Can you work these out from the model? Positions are in its coordinate system, mm. Face numbers are marked on the shaded views. A direction names the side the tool comes from. Give positions to 0.01 mm unless a question says otherwise; leave off trailing zeros. Loops run counter-clockwise (first coordinate to the right, second up) from the corner with the lowest first, then second, coordinate; pieces in that order, holes last. Notation, with made-up numbers: (47, 58.25) - (70, 58.25) arc R15 ccw to (70, 85.25) - close; hole circle Ø2 at (16.25, 34). An arc over 180 degrees is marked (long way). Answer as a JSON object with one key per item and string values.
```python
from build123d import *

# Parameters (mm, degrees)
HEXAGON_DEPTH            = 5
SKETCH3_R                = 2
SCREW_POST_DEPTH         = 11
SKETCH4_R                = 2.5
BEARING_SECTION_DEPTH    = 14
SKETCH5_R                = 6.75
U_JOINT_BASE_DEPTH       = 3
U_JOINT_STANDUPS_DEPTH   = 9.5
STANDUP_ROUND_DEPTH      = 7.928203
STANDUP_ROUND_DEPTH_BACK = 7.928203
SKETCH8_R                = 1
BALL_HOLES_DEPTH         = 7.928203
BALL_HOLES_DEPTH_BACK    = 7.928203


with BuildPart() as part:
    # Sketch2 → Hexagon (new body)
    with BuildSketch(Plane.XY):
        Polygon((3.464102, -6), (6.928203, 0), (3.464102, 6), (-3.464102, 6), (-6.928203, 0), (-3.464102, -6), align=None)
    extrude(amount=HEXAGON_DEPTH)

    # Sketch3 → Screw Post (add)
    with BuildSketch(Plane.XY.offset(5)):
        Circle(SKETCH3_R)
    extrude(amount=SCREW_POST_DEPTH)

    # Sketch4 → Bearing Section (add)
    with BuildSketch(Plane(origin=(0, 0, 0), x_dir=(-1, 0, 0), z_dir=(0, 0, -1))):
        Circle(SKETCH4_R)
    extrude(amount=BEARING_SECTION_DEPTH)

    # Sketch5 → U Joint Base (add)
    with BuildSketch(Plane(origin=(0, 0, -14), x_dir=(-1, 0, 0), z_dir=(0, 0, -1))):
        Circle(SKETCH5_R)
    extrude(amount=U_JOINT_BASE_DEPTH)

    # Sketch6 → U Joint Standups (add)
    with BuildSketch(Plane(origin=(0, 0, -17), x_dir=(-1, 0, 0), z_dir=(0, 0, -1))):
        with BuildLine():
            Line((-5.771698, 3.5), (-3.75, 3.5))
            Line((-3.75, 3.5), (-3.75, -3.5))
            Line((-3.75, -3.5), (-5.771698, -3.5))
            ThreePointArc((-5.771698, -3.5), (-6.75, 0), (-5.771698, 3.5))
        make_face()
        with BuildLine():
            Line((3.75, -3.5), (3.75, 3.5))
            Line((3.75, 3.5), (5.771698, 3.5))
            ThreePointArc((5.771698, 3.5), (6.75, 0), (5.771698, -3.5))
            Line((5.771698, -3.5), (3.75, -3.5))
        make_face()
    extrude(amount=U_JOINT_STANDUPS_DEPTH)

    # Sketch7 → Standup Round (cut, two sides)
    with BuildSketch(Plane(origin=(0, 0, 0), x_dir=(0, 0, -1), z_dir=(1, 0, 0))) as standup_round_sk:
        with BuildLine():
            Line((26.5, -3.5), (26.5, 0))
            ThreePointArc((26.5, 0), (25.474874, -2.474874), (23, -3.5))
            Line((23, -3.5), (26.5, -3.5))
        make_face()
        with BuildLine():
            Line((26.5, 3.5), (23, 3.5))
            ThreePointArc((23, 3.5), (25.474874, 2.474874), (26.5, 0))
            Line((26.5, 0), (26.5, 3.5))
        make_face()
    extrude(amount=STANDUP_ROUND_DEPTH, mode=Mode.SUBTRACT)
    extrude(standup_round_sk.sketch, amount=-STANDUP_ROUND_DEPTH_BACK, mode=Mode.SUBTRACT)

    # Sketch8 → Ball Holes (cut, two sides)
    with BuildSketch(Plane(origin=(0, 0, 0), x_dir=(0, 0, -1), z_dir=(1, 0, 0))) as ball_holes_sk:
        with Locations((23, 0)):
            Circle(SKETCH8_R)
    extrude(amount=BALL_HOLES_DEPTH, mode=Mode.SUBTRACT)
    extrude(ball_holes_sk.sketch, amount=-BALL_HOLES_DEPTH_BACK, mode=Mode.SUBTRACT)


solid = part.part
```
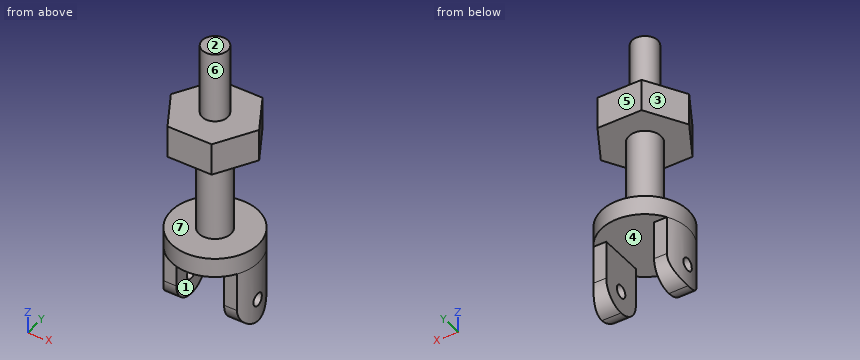
1) I need wall thicknesses on L1, parallel to Z at x = -4.9, y = 0; L2, parallel to Y at x = -4.45, z = -23; L3, parallel to Z at x = -3.5, y = -1.25. Which ranges of each line are inside material? Lowest first, please.
Check sheet entries:
{"L1": "-26.5 to -24, -22 to -14, 0 to 5", "L2": "-3.5 to -1, 1 to 3.5", "L3": "-17 to -14, 0 to 5"}
2) Imagine slicing it at D-D on z = -22.5. Write out the boundary of the cut face in (x, y).
Check sheet entries:
{"outline": "(-6.69, -0.87) arc R6.75 ccw to (-5.77, -3.5) - (-3.75, -3.5) - (-3.75, -0.87) - close; (-6.69, 0.87) - (-3.75, 0.87) - (-3.75, 3.5) - (-5.77, 3.5) arc R6.75 ccw to start; (3.75, -3.5) - (5.77, -3.5) arc R6.75 ccw to (6.69, -0.87) - (3.75, -0.87) - close; (3.75, 0.87) - (6.69, 0.87) arc R6.75 ccw to (5.77, 3.5) - (3.75, 3.5) - close"}
3) If we mould it in two halves opening along X, with no side actions, what happens to the marked faces 1, 2, 3 and 4? For each: released by +X, released by -X, zero draft, split by the parting line, or undercut.
Check sheet entries:
{"face 1": "undercut", "face 2": "zero draft", "face 3": "released by -X", "face 4": "undercut"}
4) Imagine slicing it at C-C on y = 4.25. Write out the boundary of the cut face in (x, z).
Check sheet entries:
{"outline": "(-5.24, -17) - (5.24, -17) - (5.24, -14) - (-5.24, -14) - close; (-4.47, 0) - (4.47, 0) - (4.47, 5) - (-4.47, 5) - close"}
5) Which directions (+Z, -Z, +X, -X, +Y, -Y) give clear straight access to the entire face, cutting with the end or side of a thin tool? Please do the marked faces 5, 6 and 7.
Check sheet entries:
{"face 5": "+Z, +X, -X, +Y", "face 6": "+Z", "face 7": "none"}
6) Imagine slicing it at B-B on x = 4.75. Write out the boundary of the cut face in (y, z), and give its area (3 significant figures).
Check sheet entries:
{"outline": "(-4.8, -17) - (-3.5, -17) - (-3.5, -23) arc R3.5 ccw to (0, -26.5) arc R3.5 ccw to (3.5, -23) - (3.5, -17) - (4.8, -17) - (4.8, -14) - (-4.8, -14) - close; (-3.77, 0) - (3.77, 0) - (3.77, 5) - (-3.77, 5) - close; hole circle Ø2 at (0, -23)", "area": "125 mm2"}
7) I'm going to push flat-ended pins straight in: P1, Ø4, axis at x = 2, y = 5.5, coming from the -Z side; P2, Ø2, axis at x = -2.5, y = -2, coming from the +Z side; P3, Ø2.5, axis at y = 0, z = -23, coming from the -X side. Where does each tip first touch, or does it pass through?
Check sheet entries:
{"P1": "z = -17", "P2": "z = 5", "P3": "x = -6.75"}
8) Imagine slicing it at A-A on z = -18. Write out the boundary of the cut face in (x, y), and give its area (3 significant figures).
Check sheet entries:
{"outline": "(-5.77, -3.5) - (-3.75, -3.5) - (-3.75, 3.5) - (-5.77, 3.5) arc R6.75 ccw to start; (3.75, -3.5) - (5.77, -3.5) arc R6.75 ccw to (5.77, 3.5) - (3.75, 3.5) - close", "area": "37.6 mm2"}
